```python
from build123d import *

# Parameters (mm, degrees)
PAD_DEPTH       = 18
SKETCH001_R     = 3
POCKET_DEPTH    = 39.7525374288
SKETCH002_R     = 3
POCKET001_DEPTH = 29.7259431815
CHAMFER_SIZE    = 1


with BuildPart() as part:
    # Sketch → Pad (new body)
    with BuildSketch(Plane.XY):
        Polygon((-8.2819133905, -13), (-20.9604612427, 14.1892336111), (-15.5226145205, 16.7249431815), (-4.4594918257, -7), (21.7180866095, -7), (21.7180866095, -13), align=None)
    extrude(amount=PAD_DEPTH)

    # Sketch001 (on Face1 of Pad) → Pocket (cut, through all)
    with BuildSketch(Plane(origin=(-11.7820012315, -5.4940374026, 0), x_dir=(0.4226182617, -0.906307787, 0), z_dir=(-0.906307787, -0.4226182617, 0))):
        with Locations((-15.7180866095, 9)):
            Circle(SKETCH001_R)
    extrude(amount=-POCKET_DEPTH, mode=Mode.SUBTRACT)

    # Sketch002 (on Face2 of Pocket) → Pocket001 (cut, through all)
    with BuildSketch(Plane.XZ.offset(13)):
        with Locations((15.7180866095, 9)):
            Circle(SKETCH002_R)
    extrude(amount=-POCKET001_DEPTH, mode=Mode.SUBTRACT)

    # Chamfer
    chamfer_edges = [part.edges().sort_by_distance(p)[0] for p in [
        (-14.621187, 0.594617, 18),
        (-18.241538, 15.457088, 18),
        (-9.991053, 4.862472, 18),
        (8.629297, -7, 18),
        (21.718087, -10, 18),
        (6.718087, -13, 18),
        (-14.621187, 0.594617, 0),
        (-18.241538, 15.457088, 0),
        (-9.991053, 4.862472, 0),
        (8.629297, -7, 0),
        (21.718087, -10, 0),
        (6.718087, -13, 0),
    ]]
    chamfer(chamfer_edges, length=CHAMFER_SIZE)


solid = part.part
```
CAD build for the part. Positions are in the model's coordinates, mm. A direction names the side the tool comes from. Round coordinates to 2 decimals unless told otherwise and drop trailing zeros. Order: outer loops, then holes, each group sorted by start corner. A loop starts at its lowest first (then second) coordinate and runs counter-clockwise, first axis right, second up.
Q1. Which spindle directions (+Z, -Z, +X, -X, +Y, -Y) get a long thin tool onto all of the face, cutting with end or side? Do faces 5 (the flat face through (8.1, -7.5, 17.5)), 6 (the flat face through (8.1, -7.5, 0.5)), 7 (the flat face through (-18.071, 14.993, 17.493)). Say none if no direction does.
Q2. Slice it at B-B (x = 18). Write the cut outline in (y, z), and give its area (3 significant figures).
Q3. Slice it at A-A (z = 10.25). Write the cut outline in (x, y), and give its area (3 significant figures).
Q4. Wall check: L1, parallel to Y at x = 11, z = 1.25; L2, parallel to Z at x = -15.5, y = 10.75; L3, parallel to Z at x = -15, y = 7.5. Give the ranges that are in metal, low to high.
Q5. Drop flat-ended pins along their axis: pin 1 (7 mm diameter, centred on x = 15.72, z = 9, fed in from +Y); pin 2 (5 mm diameter, centred on y = 6.5, z = 2.5, fed in from +X); pin 3 (5 mm diameter, centred on y = -2.5, z = 7.5, fed in from +X). Give the stop position or say it passes through.
Q6. Slice it at C-C (x = 0.5). Write the cut outline in (y, z), and give its area (3 significant figures).
Q7. Slice it at D-D (y = 2). Write the cut outline in (x, z), and give its area (3 significant figures).
Q8. Two-plate mould, pull along Z, no slides. Class faces 1 (the cylindrical face through (-15.159, 8.747, 6.338)), 2 (the flat face through (6.9, -12.5, 0.5)), 3 (the cylindrical face through (12.72, -10.04, 9.13)), 4 (the flat face through (8, -7, 9)): pulls with the +Z half, pulls with the -Z half, needs draft (parallel to the pull), parting line crosses it, or undercut.
Results below:
1. face 5: +Z, +X, +Y
1. face 6: -Z, +X, +Y
1. face 7: +Z, -X, +Y
2. outline: (-13, 1) - (-12, 0) - (-8, 0) - (-7, 1) - (-7, 7.05) - (-13, 7.05) - close; (-13, 10.95) - (-7, 10.95) - (-7, 17) - (-8, 18) - (-12, 18) - (-13, 17) - close
2. area: 82.6 mm2
3. outline: (-20.96, 14.19) - (-19.58, 11.22) - (-14.14, 13.76) - (-15.52, 16.72) - close; (-17.27, 6.28) - (-8.28, -13) - (12.99, -13) - (12.99, -7) - (-4.46, -7) - (-11.83, 8.82) - close; (18.45, -13) - (21.72, -13) - (21.72, -7) - (18.45, -7) - close
3. area: 272 mm2
4. L1: y = -13 to -7
4. L2: z = 0 to 6.06, 11.94 to 18
4. L3: z = 0 to 7.47, 10.53 to 18
5. pin 1: stops at y = -7
5. pin 2: stops at x = -9.59
5. pin 3: stops at x = -5.39
6. outline: (-13, 1) - (-12, 0) - (-8, 0) - (-7, 1) - (-7, 17) - (-8, 18) - (-12, 18) - (-13, 17) - close
6. area: 106 mm2
7. outline: (-15.28, 1) - (-14.17, 0) - (-9.76, 0) - (-8.66, 1) - (-8.66, 17) - (-9.76, 18) - (-14.17, 18) - (-15.28, 17) - close
7. area: 117 mm2
8. face 1: undercut
8. face 2: pulls with the -Z half
8. face 3: undercut
8. face 4: needs draft
